```python
from build123d import *

# Parameters (mm, degrees)
F0_R     = 1.27
F1_DEPTH = 1.651


with BuildPart() as f1:
    # F0 (on Top) → F1 (new body)
    with BuildSketch(Plane.XY):
        with BuildLine():
            Line((-15.1765, -18.2245), (15.1765, -18.2245))
            ThreePointArc((15.1765, -18.2245), (16.972551, -17.480551), (17.7165, -15.6845))
            Line((17.7165, -15.6845), (17.7165, -15.0495))
            Line((17.7165, -15.0495), (20.8915, -15.0495))
            Line((20.8915, -15.0495), (20.8915, 15.0495))
            Line((20.8915, 15.0495), (17.7165, 15.0495))
            Line((17.7165, 15.0495), (17.7165, 15.6845))
            ThreePointArc((17.7165, 15.6845), (16.972551, 17.480551), (15.1765, 18.2245))
            Line((15.1765, 18.2245), (-15.1765, 18.2245))
            ThreePointArc((-15.1765, 18.2245), (-16.972551, 17.480551), (-17.7165, 15.6845))
            Line((-17.7165, 15.6845), (-17.7165, 15.0495))
            Line((-17.7165, 15.0495), (-20.8915, 15.0495))
            Line((-20.8915, 15.0495), (-20.8915, 4.0005))
            Line((-20.8915, 4.0005), (-17.7165, 4.0005))
            Line((-17.7165, 4.0005), (-17.7165, -4.0005))
            Line((-17.7165, -4.0005), (-20.8915, -4.0005))
            Line((-20.8915, -4.0005), (-20.8915, -15.0495))
            Line((-20.8915, -15.0495), (-17.7165, -15.0495))
            Line((-17.7165, -15.0495), (-17.7165, -15.6845))
            ThreePointArc((-17.7165, -15.6845), (-16.972551, -17.480551), (-15.1765, -18.2245))
        make_face()
        with Locations((-15.24, -15.24)):
            Circle(F0_R, mode=Mode.SUBTRACT)
        with Locations((15.24, -15.24)):
            Circle(F0_R, mode=Mode.SUBTRACT)
        with Locations((-15.24, 15.24)):
            Circle(F0_R, mode=Mode.SUBTRACT)
        with Locations((15.24, 15.24)):
            Circle(F0_R, mode=Mode.SUBTRACT)
    extrude(amount=F1_DEPTH)


solid = f1.part
```
Geometry: final body of the model. Coordinates: model frame, mm. A direction names the side the tool comes from. Round coordinates to 2 decimals unless told otherwise and drop trailing zeros. Loops run counter-clockwise (first coordinate to the right, second up) from the corner with the lowest first, then second, coordinate; pieces in that order, holes last. Notation, with made-up numbers: (50, 9.5) -> (86, 9.5) arc R16 ccw to (86, 31.5) -> close; hole circle Ø4 at (86.25, -38.5). An arc over 180 degrees is marked (long way). Use one line per item in the form item = value.
Item 1: Cut plane A-A on z = 0.9. Output: boundary loops of the cut face in (x, y), then the cut area to 3 significant figures.
Evaluation:
outline = (-20.89, -15.05) -> (-17.72, -15.05) -> (-17.72, -15.68) arc R2.54 ccw to (-15.18, -18.22) -> (15.18, -18.22) arc R2.54 ccw to (17.72, -15.68) -> (17.72, -15.05) -> (20.89, -15.05) -> (20.89, 15.05) -> (17.72, 15.05) -> (17.72, 15.68) arc R2.54 ccw to (15.18, 18.22) -> (-15.18, 18.22) arc R2.54 ccw to (-17.72, 15.68) -> (-17.72, 15.05) -> (-20.89, 15.05) -> (-20.89, 4) -> (-17.72, 4) -> (-17.72, -4) -> (-20.89, -4) -> close; hole circle Ø2.54 at (-15.24, -15.24); hole circle Ø2.54 at (-15.24, 15.24); hole circle Ø2.54 at (15.24, -15.24); hole circle Ø2.54 at (15.24, 15.24)
area = 1,430 mm2
Item 2: Material intervals for probe 1 along Y at (x, z) = (15.24, 1.25); probe 2 along Y at (x, z) = (17, 1.5), sorted ascending.
Evaluation:
probe_1 = -18.22 to -16.51, -13.97 to 13.97, 16.51 to 18.22
probe_2 = -17.45 to 17.45
Item 3: Cut plane B-B on y = -14.5. Output: boundary loops of the cut face in (x, z), then the cut area to 3 significant figures.
Evaluation:
outline = (-20.89, 0) -> (-16.27, 0) -> (-16.27, 1.65) -> (-20.89, 1.65) -> close; (-14.21, 0) -> (14.21, 0) -> (14.21, 1.65) -> (-14.21, 1.65) -> close; (16.27, 0) -> (20.89, 0) -> (20.89, 1.65) -> (16.27, 1.65) -> close
area = 62.2 mm2
Item 4: Contact query for flat-ended pins moving along their axis: pin 1 Ø0.7 at (y, z) = (15.5, 1) entering from -X; pin 2 Ø0.5 at (y, z) = (-15.5, 1) entering from +X; pin 3 Ø2 at (x, y) = (-8.5, 7.5) entering from -Z; pin 4 Ø0.8 at (x, z) = (19.5, 0.5) entering from +Y. Output: stop coordinate, or through.
Evaluation:
pin_1 = -17.72
pin_2 = 17.72
pin_3 = 0
pin_4 = 15.05
Item 5: Draft query along Y for faces 4 (the cylindrical face through (-15.41, -13.98, 0.81)), 5 (the flat face through (-20.892, -9, 1)), 6 (the flat face through (19, -15.05, 1)). Return one class per face: released by +Y, released by -Y, zero draft, split by the parting line, or undercut.
Evaluation:
face_4 = undercut
face_5 = zero draft
face_6 = released by -Y
Item 6: Access query for faces 1 (the flat face through (-19, -15.05, 1)), 2 (the flat face through (-19, -4, 1)), 3 (the flat face through (19, 15.05, 1)). Directions: +Z, -Z, +X, -X, +Y, -Y. A direction counts if a zero-diameter tool reaches every point of the face in a straight line with its end or side. Return the directions, or none.
Evaluation:
face_1 = +Z, -Z, -X, -Y
face_2 = +Z, -Z, -X
face_3 = +Z, -Z, +X, +Y
